```python
from build123d import *

# Parameters (mm, degrees)
F1_DEPTH = 3.175


# Not quite as in the source:
# - a length typed as a fraction of an inch, garbled in the dataset ("3 / 203.2 mm" for 3/8 in), is restored


with BuildPart() as f1:
    # F0 (on Top) → F1 (new body)
    with BuildSketch(Plane.XY):
        Polygon((84.4656275958, 81.8700266516), (-45.5343724042, 81.8700266516), (-65.5343724042, 61.8700266516), (-30.5343724042, 31.8700266516), (-65.5343724042, 1.8700266516), (-45.5343724042, -18.1299733484), (84.4656275958, -18.1299733484), (104.4656275958, 1.8700266516), (104.4656275958, 61.8700266516), align=None)
        Polygon((-15.5343724042, -12.9424554378), (-15.5343724042, 2.0575445622), (3.6249275958, 2.0575445622), (3.6249275958, 5.2325445622), (14.0516275958, 5.2325445622), (14.0516275958, 2.0575445622), (34.8796275958, 2.0575445622), (34.8796275958, 5.2325445622), (45.3063275958, 5.2325445622), (45.3063275958, 2.0575445622), (64.4656275958, 2.0575445622), (74.4656275958, 2.0575445622), (79.4656275958, 2.0575445622), (79.4656275958, -12.9424554378), (74.4656275958, -12.9424554378), (64.4656275958, -12.9424554378), (45.3063275958, -12.9424554378), (45.3063275958, -16.1174554378), (34.8796275958, -16.1174554378), (34.8796275958, -12.9424554378), (14.0516275958, -12.9424554378), (14.0516275958, -16.1174554378), (3.6249275958, -16.1174554378), (3.6249275958, -12.9424554378), align=None, mode=Mode.SUBTRACT)
        Polygon((-15.5343724042, 61.8700266516), (-15.5343724042, 76.8700266516), (3.6249275958, 76.8700266516), (3.6249275958, 80.0450266516), (14.0516275958, 80.0450266516), (14.0516275958, 76.8700266516), (34.8796275958, 76.8700266516), (34.8796275958, 80.0450266516), (45.3063275958, 80.0450266516), (45.3063275958, 76.8700266516), (64.4656275958, 76.8700266516), (74.4656275958, 76.8700266516), (79.4656275958, 76.8700266516), (79.4656275958, 61.8700266516), (74.4656275958, 61.8700266516), (64.4656275958, 61.8700266516), (45.3063275958, 61.8700266516), (45.3063275958, 58.6950266516), (34.8796275958, 58.6950266516), (34.8796275958, 61.8700266516), (14.0516275958, 61.8700266516), (14.0516275958, 58.6950266516), (3.6249275958, 58.6950266516), (3.6249275958, 61.8700266516), align=None, mode=Mode.SUBTRACT)
    extrude(amount=F1_DEPTH)


solid = f1.part
```
CAD build for the part. Positions are in the model's coordinates, mm. Coordinates: 2 decimals unless noted, no trailing zeros. Write each loop counter-clockwise with the first axis right and the second up, starting at its lowest first coordinate (ties: lowest second). Pieces come first, ordered by that corner, then holes.
(1) Cut at C-C, the plane x = -51. List the corners of the cut face in (y, z) (3 decimals).
(2) Cut at D-D, the plane z = 1.8. Count the separate pieces of the cut face and the enclosed holes in it, and give its area (3 significant figures).
(3) Flat gauge pins, fed straight in: pin 1 (1.6 mm diameter, centred on y = 70.5, z = 2.5, fed in from +X); pin 2 (1.6 mm diameter, centred on y = -2, z = 2, fed in from +X); pin 3 (1.5 mm diameter, centred on y = 15.5, z = 1, fed in from -X). Where does each tip first touch, or does it go through?
(4) Cut at B-B, the plane y = 72. List the corners of the cut face in (x, z) (3 decimals), and give its area (3 significant figures).
(5) Cut at A-A, the plane x = 54.5. List the corners of the cut face in (y, z) (3 decimals), and give its area (3 significant figures).
(6) Drill centre lines: probe 1 along Y at (x, z) = (-13, 2.7); probe 2 along Y at (x, z) = (9.5, 2.35); probe 3 along X at (y, z) = (-9, 0.85). Where is each one in solid material? Low to high.
(7) Two-plate mould, pull along X, no slides. Class faces 1 (the face through (-15.534, 69, 2)), 2 (the face through (18, 33, 0)): +X half, -X half, draft (parallel to the pull), parting line (faces both ways), or undercut.
Geometry says:
1. outline: (-12.664, 0) - (14.328, 0) - (14.328, 3.175) - (-12.664, 3.175) - close; (49.412, 0) - (76.404, 0) - (76.404, 3.175) - (49.412, 3.175) - close
2. separate pieces: 1
2. enclosed holes: 2
2. area: 12,000 mm2
3. pin 1: stops at x = 96.64
3. pin 2: stops at x = 101.4
3. pin 3: stops at x = -50.51
4. outline: (-55.404, 0) - (-15.534, 0) - (-15.534, 3.175) - (-55.404, 3.175) - close; (79.466, 0) - (94.336, 0) - (94.336, 3.175) - (79.466, 3.175) - close
4. area: 174 mm2
5. outline: (-18.13, 0) - (-12.942, 0) - (-12.942, 3.175) - (-18.13, 3.175) - close; (2.058, 0) - (61.87, 0) - (61.87, 3.175) - (2.058, 3.175) - close; (76.87, 0) - (81.87, 0) - (81.87, 3.175) - (76.87, 3.175) - close
5. area: 222 mm2
6. probe 1: y = -18.13 to -12.94, 2.06 to 61.87, 76.87 to 81.87
6. probe 2: y = -18.13 to -16.12, 5.23 to 58.7, 80.05 to 81.87
6. probe 3: x = -54.66 to -15.53, 79.47 to 93.6
7. face 1: undercut
7. face 2: draft
